```python
from build123d import *

# Parameters (mm, degrees)
SKETCH1_R           = 14.2875
SKETCH1_R_2         = 3.3734375
SKETCH1_R_3         = 2.5527
BOSS_EXTRUDE1_DEPTH = 6.35


with BuildPart() as part:
    # Sketch1 → Boss-Extrude1 (new body)
    with BuildSketch(Plane.XY):
        with BuildLine():
            Line((-93.6625, -38.1), (93.6625, -38.1))
            ThreePointArc((93.6625, -38.1), (99.275160076, -35.775160076), (101.6, -30.1625))
            Line((101.6, -30.1625), (101.6, 30.1625))
            ThreePointArc((101.6, 30.1625), (99.275160076, 35.775160076), (93.6625, 38.1))
            Line((93.6625, 38.1), (-93.6625, 38.1))
            ThreePointArc((-93.6625, 38.1), (-99.275160076, 35.775160076), (-101.6, 30.1625))
            Line((-101.6, 30.1625), (-101.6, -30.1625))
            ThreePointArc((-101.6, -30.1625), (-99.275160076, -35.775160076), (-93.6625, -38.1))
        make_face()
        Circle(SKETCH1_R, mode=Mode.SUBTRACT)
        with Locations((52.5018, 0)):
            Circle(SKETCH1_R, mode=Mode.SUBTRACT)
        with Locations((-93.6625, 30.1625)):
            Circle(SKETCH1_R_2, mode=Mode.SUBTRACT)
        with Locations((93.6625, 30.1625)):
            Circle(SKETCH1_R_2, mode=Mode.SUBTRACT)
        with Locations((93.6625, -30.1625)):
            Circle(SKETCH1_R_2, mode=Mode.SUBTRACT)
        with Locations((-93.6625, -30.1625)):
            Circle(SKETCH1_R_2, mode=Mode.SUBTRACT)
        with Locations((-52.5018, 25.4)):
            Circle(SKETCH1_R_3, mode=Mode.SUBTRACT)
        with Locations((-52.5018, -25.4)):
            Circle(SKETCH1_R_3, mode=Mode.SUBTRACT)
        with BuildLine():
            Line((-28.601593607, 4.3688), (-27.1018, 4.3688))
            ThreePointArc((-27.1018, 4.3688), (-22.733, 0), (-27.1018, -4.3688))
            Line((-27.1018, -4.3688), (-28.601593607, -4.3688))
            ThreePointArc((-28.601593607, -4.3688), (-32.052828476, -5.388558178), (-34.395583036, -8.12030303))
            ThreePointArc((-34.395583036, -8.12030303), (-52.5018, -19.84375), (-70.608016964, -8.12030303))
            ThreePointArc((-70.608016964, -8.12030303), (-72.950771524, -5.388558178), (-76.402006393, -4.3688))
            Line((-76.402006393, -4.3688), (-77.9018, -4.3688))
            ThreePointArc((-77.9018, -4.3688), (-82.2706, 0), (-77.9018, 4.3688))
            Line((-77.9018, 4.3688), (-76.402006393, 4.3688))
            ThreePointArc((-76.402006393, 4.3688), (-72.950771524, 5.388558178), (-70.608016964, 8.12030303))
            ThreePointArc((-70.608016964, 8.12030303), (-52.5018, 19.84375), (-34.395583036, 8.12030303))
            ThreePointArc((-34.395583036, 8.12030303), (-32.052828476, 5.388558178), (-28.601593607, 4.3688))
        make_face(mode=Mode.SUBTRACT)
    extrude(amount=BOSS_EXTRUDE1_DEPTH)


solid = part.part
```
Geometry check sheet. Reference: the model listing, model coordinates, mm. A direction names the side the tool comes from. Round coordinates to 2 decimals unless told otherwise and drop trailing zeros. Write each loop counter-clockwise with the first axis right and the second up, starting at its lowest first coordinate (ties: lowest second). Pieces come first, ordered by that corner, then holes. Notation, with made-up numbers: (12, 60.25) - (34, 60.25) arc R22 cw to (34, 93.25) - close; hole circle Ø5 at (46, 79.5). An arc over 180 degrees is marked (long way). Write each question's results on one line, items separated by ' | '.
(1) Set-up check for faces 1 (the face through (-32.01, -5.36, 3.13)), 2 (the face through (-99.34, -35.71, 3.13)): record each of +Z, -Z, +X, -X, +Y, -Y from which the full face is reachable in a straight line by a thin tool's end or side.
Computed:
face 1: +Z, -Z | face 2: +Z, -Z, -X, -Y
(2) Sectioned sample at C-C, the plane x = 0. Enter the section's corners in (y, z), plus the area to 3 significant figures.
Computed:
outline: (-38.1, 0) - (-14.29, 0) - (-14.29, 6.35) - (-38.1, 6.35) - close; (14.29, 0) - (38.1, 0) - (38.1, 6.35) - (14.29, 6.35) - close | area: 302 mm^2
(3) Sectioned sample at B-B, the plane z = 4.25. Count the separate pieces of the cut face and the enclosed holes in it, plus the area to 3 significant figures.
Computed:
separate pieces: 1 | enclosed holes: 9 | area: 12,600 mm^2
(4) Draft check along X on faces 3 (the face through (99.21, -35.84, 3.13)), 4 (the face through (-99.21, 35.84, 3.13)), 5 (the face through (-14.274, 0.628, 3.131)). Enter one of: pulls with the +X half, pulls with the -X half, needs draft (parallel to the pull), parting line crosses it, or undercut.
Computed:
face 3: pulls with the +X half | face 4: pulls with the -X half | face 5: undercut
(5) Depth check by flat-ended pin: pin 1 Ø8 at (x, y) = (80.5, 18.5) entering from -Z; pin 2 Ø6 at (x, y) = (93.66, 30.16) entering from -Z. Enter the tip coordinate at first touch or a pass-through.
Computed:
pin 1: stops at z = 0 | pin 2: passes through
(6) Sectioned sample at A-A, the plane y = 0. Enter the section's corners in (x, z).
Computed:
outline: (-101.6, 0) - (-82.27, 0) - (-82.27, 6.35) - (-101.6, 6.35) - close; (-22.73, 0) - (-14.29, 0) - (-14.29, 6.35) - (-22.73, 6.35) - close; (14.29, 0) - (38.21, 0) - (38.21, 6.35) - (14.29, 6.35) - close; (66.79, 0) - (101.6, 0) - (101.6, 6.35) - (66.79, 6.35) - close
(7) Sectioned sample at D-D, the plane x = -43. Enter the section's corners in (y, z), plus the area to 3 significant figures.
Computed:
outline: (-38.1, 0) - (-17.42, 0) - (-17.42, 6.35) - (-38.1, 6.35) - close; (17.42, 0) - (38.1, 0) - (38.1, 6.35) - (17.42, 6.35) - close | area: 263 mm^2
(8) Thickness scan on probe 1 along X at (y, z) = (30, 4); probe 2 along X at (y, z) = (33, 2); probe 3 along Y at (x, z) = (0, 4). Record the ranges inside material, lowest first. Write a range as from..to.
Computed:
probe 1: x = -101.6..-97.03, -90.29..90.29, 97.03..101.6 | probe 2: x = -101.08..-95.49, -91.84..91.84, 95.49..101.08 | probe 3: y = -38.1..-14.29, 14.29..38.1
